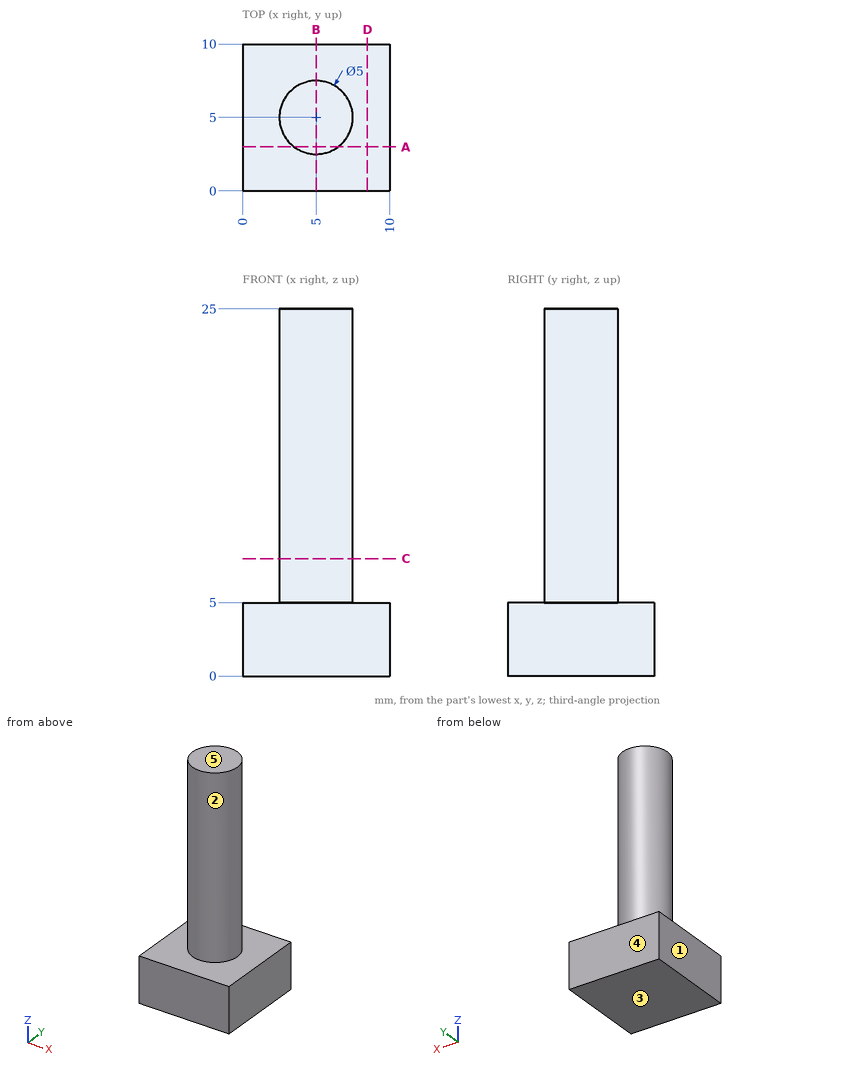
Geometry check sheet. Reference: drawing and pictorial views, mm from the part's lowest x, y, z. A direction names the side the tool comes from. Coordinates: 2 decimals unless noted, no trailing zeros. Write each loop counter-clockwise with the first axis right and the second up, starting at its lowest first coordinate (ties: lowest second). Pieces come first, ordered by that corner, then holes. Notation, with made-up numbers: M -28,51 L 15,51 A16 ccw 15,75 Z; hole C 37.25,3.5 d11. An arc over 180 degrees is marked long. Use one line per item in the form item = value.
Item 1: Set-up check for the marked faces 1 and 2: record each of +Z, -Z, +X, -X, +Y, -Y from which the full face is reachable in a straight line by a thin tool's end or side.
Answer below:
face_1 = +Z, -Z, -X, +Y, -Y
face_2 = +Z
Item 2: Sectioned sample at C-C, the plane z = 8. Record the cut outline in (x, y), and give its area (3 significant figures).
Answer below:
outline = C 5,5 d5
area = 19.6 mm^2
Item 3: Gauge pin test, flat ends, axial feed: pin 1 Ø5 at (y, z) = (7.5, 14.5) entering from -X; pin 2 Ø5 at (x, z) = (4.5, 18) entering from +Y; pin 3 Ø1.5 at (x, z) = (3.5, 9.5) entering from -Y; pin 4 Ø1 at (x, y) = (4, 9) entering from -Z. Record the tip position at first contact, or that the pin passes through.
Answer below:
pin_1 = 2.5
pin_2 = 7.5
pin_3 = 2.62
pin_4 = 0
Item 4: Sectioned sample at D-D, the plane x = 8.5. Record the cut outline in (y, z).
Answer below:
outline = M 0,0 L 10,0 L 10,5 L 0,5 Z
Item 5: Sectioned sample at A-A, the plane y = 3. Record the cut outline in (x, z).
Answer below:
outline = M 0,0 L 10,0 L 10,5 L 6.5,5 L 6.5,25 L 3.5,25 L 3.5,5 L 0,5 Z
Item 6: Release check for a two-part mould opening along Z. For the marked faces 3, 4 and 5 record: pulls with the +Z half, pulls with the -Z half, needs draft (parallel to the pull), parting line crosses it, or undercut.
Answer below:
face_3 = pulls with the -Z half
face_4 = needs draft
face_5 = pulls with the +Z half
Item 7: Material ranges on L1, parallel to Z at x = 5.75, y = 9.5; L2, parallel to Y at x = 7, z = 18.5; L3, parallel to X at y = 4.5, z = 17.25, recorded low to high. Write a range as from..to.
Answer below:
L1 = 0..5
L2 = 3.5..6.5
L3 = 2.55..7.45
Item 8: Sectioned sample at B-B, the plane x = 5. Record the cut outline in (y, z), and give its area (3 significant figures).
Answer below:
outline = M 0,0 L 10,0 L 10,5 L 7.5,5 L 7.5,25 L 2.5,25 L 2.5,5 L 0,5 Z
area = 150 mm^2
